Input: part model. Units: mm. Frame: model coordinates. Face numbers are marked on the shaded views. A direction names the side the tool comes from. Coordinates: 2 decimals unless noted, no trailing zeros. Loops run counter-clockwise (first coordinate to the right, second up) from the corner with the lowest first, then second, coordinate; pieces in that order, holes last.
Item 1: Ray query, line 1 along Y through (x, z) = (0, 3.25); line 2 along Y through (x, z) = (0, 11.5); line 3 along Z through (x, y) = (-2, 3.25). Return the intervals inside material, ascending.
Item 2: Contact query for flat-ended pins moving along their axis: P1, Ø6, axis at x = 4, z = 0, coming from the -Y side; P2, Ø6, axis at x = 1.5, y = -4.5, coming from the +Z side; P3, Ø6, axis at x = 4.5, z = 10, coming from the -Y side. Output: stop coordinate, or through.
Item 3: Section D-D on y = -3. Return loops of the section in (x, z).
Item 4: Reachability of the marked faces 1 and 2 from +Z, -Z, +X, -X, +Y, -Y: full face, straight path, thin tool, end or side. Return the list, or none.
Item 5: Pull-direction query (X, two-part tool) for the marked faces 3, 4 and 5; classes: released by +X, released by -X, zero draft, split by the parting line, or undercut.
Item 6: Section A-A on y = 0. Return loops of the section in (x, z).
Item 7: Section C-C on z = 10. Return loops of the section in (x, y), and give its area (3 significant figures).
```python
from build123d import *

# Parameters (mm, degrees)
F0_R     = 3.95
F1_DEPTH = 8
F2_R     = 2.6
F3_DEPTH = 7
F4_SIZE  = 1
F5_R     = 6
F6_DEPTH = 2
F7_R     = 1.5
F8_DEPTH = 17.001


with BuildPart() as f1:
    # F0 (on Top) → F1 (new body)
    with BuildSketch(Plane.XY):
        Circle(F0_R)
    extrude(amount=F1_DEPTH)

    # F2 (on face) → F3 (join)
    with BuildSketch(Plane.XY.offset(8)):
        Circle(F2_R)
    extrude(amount=F3_DEPTH)

    # F4
    f4_edges = [f1.edges().sort_by_distance(p)[0] for p in [
        (-2.6, 0, 15),
    ]]
    chamfer(f4_edges, length=F4_SIZE)

    # F5 (on face) → F6 (join)
    with BuildSketch(Plane(origin=(0, 0, 0), x_dir=(1, 0, 0), z_dir=(0, 0, -1))):
        Circle(F5_R)
    extrude(amount=F6_DEPTH)

    # F7 (on face) → F8 (cut, through all)
    with BuildSketch(Plane(origin=(0, 0, -2), x_dir=(1, 0, 0), z_dir=(0, 0, -1))):
        Circle(F7_R)
    extrude(amount=-F8_DEPTH, mode=Mode.SUBTRACT)


solid = f1.part
```
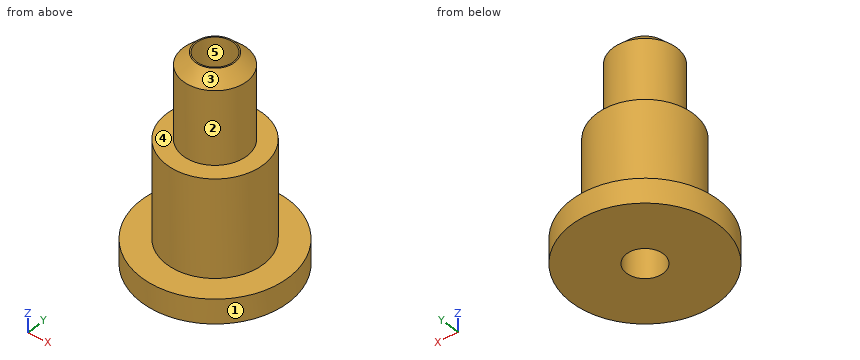
Results found:
1. line 1: y = -3.95 to -1.5, 1.5 to 3.95
1. line 2: y = -2.6 to -1.5, 1.5 to 2.6
1. line 3: z = -2 to 8
2. P1: stops at y = -5.92
2. P2: stops at z = 14.86
2. P3: stops at y = -3.24
3. outline: (-5.2, -2) - (5.2, -2) - (5.2, 0) - (2.57, 0) - (2.57, 8) - (-2.57, 8) - (-2.57, 0) - (-5.2, 0) - close
4. face 1: +Z, -Z
4. face 2: +Z
5. face 3: split by the parting line
5. face 4: zero draft
5. face 5: undercut
6. outline: (-6, -2) - (-1.5, -2) - (-1.5, 15) - (-1.6, 15) - (-2.6, 14) - (-2.6, 8) - (-3.95, 8) - (-3.95, 0) - (-6, 0) - close; (1.5, -2) - (6, -2) - (6, 0) - (3.95, 0) - (3.95, 8) - (2.6, 8) - (2.6, 14) - (1.6, 15) - (1.5, 15) - close
7. outline: circle Ø5.2 at (0, 0); hole circle Ø3 at (0, 0)
7. area: 14.2 mm2
